Work out the finished part from the listing and answer in its coordinate system (mm). A direction names the side the tool comes from. Give positions to 0.01 mm unless a question says otherwise; leave off trailing zeros. Loops run counter-clockwise (first coordinate to the right, second up) from the corner with the lowest first, then second, coordinate; pieces in that order, holes last.
```python
from build123d import *

# Parameters (mm, degrees)
RESSALTO_EXTRUS_O2_DEPTH = 30
ESBO_O5_R                = 6
CORTE_EXTRUS_O1_DEPTH    = 30


with BuildPart() as part:
    # Esboço3 → Ressalto-extrusão2 (new body)
    with BuildSketch(Plane(origin=(0, 0, 0), x_dir=(0, 0, -1), z_dir=(1, 0, 0))):
        with BuildLine():
            Line((42.248831229, -47.335013165), (42.248831229, 2.664986835))
            Line((42.248831229, 2.664986835), (32.248831229, 2.664986835))
            Line((32.248831229, 2.664986835), (32.248831229, -1.335013165))
            ThreePointArc((32.248831229, -1.335013165), (30.491471916, -5.577653852), (26.248831229, -7.335013165))
            Line((26.248831229, -7.335013165), (6.748831229, -7.335013165))
            ThreePointArc((6.748831229, -7.335013165), (-3.504217098, -11.581964838), (-7.751168771, -21.835013165))
            Line((-7.751168771, -21.835013165), (-7.751168771, -22.835013165))
            ThreePointArc((-7.751168771, -22.835013165), (-3.504217098, -33.088061493), (6.748831229, -37.335013165))
            Line((6.748831229, -37.335013165), (26.248831229, -37.335013165))
            ThreePointArc((26.248831229, -37.335013165), (30.491471916, -39.092372478), (32.248831229, -43.335013165))
            Line((32.248831229, -43.335013165), (32.248831229, -47.335013165))
            Line((32.248831229, -47.335013165), (42.248831229, -47.335013165))
        make_face()
    extrude(amount=-RESSALTO_EXTRUS_O2_DEPTH)

    # Esboço5 → Corte-extrusão1 (cut)
    with BuildSketch(Plane(origin=(0, 0, 0), x_dir=(0, 0, -1), z_dir=(1, 0, 0))):
        with Locations((6.748831229, -22.335013165)):
            Circle(ESBO_O5_R)
    extrude(amount=-CORTE_EXTRUS_O1_DEPTH, mode=Mode.SUBTRACT)


solid = part.part
```
Q1. Section C-C on x = -21 is taken. Give the vertices of the cut face in (y, z), plus the area to 3 significant figures.
Q2. Which of the six approach directions +Z, -Z, +X, -X, +Y, -Y give full straight-line access (tool end or side, diameter ignored) to faces 1 (the face through (-15, 1, -32.249)), 2 (the face through (-15, -23, -42.249)), 3 (the face through (-15, -45, -32.249))?
Q3. Section B-B on y = -17 is taken. Give the vertices of the cut face in (x, z).
Q4. Section D-D on z = -24 is taken. Give the vertices of the cut face in (x, y).
Q5. Section A-A on z = -4 is taken. Give the vertices of the cut face in (x, y), plus the area to 3 significant figures.
Q6. Given pin 1 (15.5 mm diameter, centred on x = -12.5, z = -20.5, fed in from +Y); pin 2 (2 mm diameter, centred on x = -5, z = -1.5, fed in from +Y); pin 3 (15.5 mm diameter, centred on x = -11, z = -18.5, fed in from -Y) (3 decimals), each flat-ended and moving along its own axis, determine where each tip first touches the part or whether it passes through.
Q7. Consider line 1 along Y through (x, z) = (-1.5, -9); line 2 along Y through (x, z) = (-8, -8.5); line 3 along Y through (x, z) = (-7, -20). Determine where each line is inside the solid, lowest interval first.
Q8. Determine the mould class of faces 4 (the face through (-15, -47.335, -37)), 5 (the face through (-30, -22, -22)), 6 (the face through (-15, -7.335, -17)), 7 (the face through (-14.79, -17.276, -9.974)) for opening direction Y: +Y half, -Y half, draft (parallel to the pull), parting line (faces both ways), or undercut.
Check result:
1. outline: (-47.34, -42.25) - (2.66, -42.25) - (2.66, -32.25) - (-1.34, -32.25) arc R6 cw to (-7.34, -26.25) - (-7.34, -6.75) arc R14.5 ccw to (-21.84, 7.75) - (-22.84, 7.75) arc R14.5 ccw to (-37.34, -6.75) - (-37.34, -26.25) arc R6 cw to (-43.34, -32.25) - (-47.34, -32.25) - close; hole circle Ø12 at (-22.34, -6.75)
1. area: 1,510 mm2
2. face 1: +Z, +X, -X, +Y
2. face 2: -Z, +X, -X, +Y, -Y
2. face 3: +Z, +X, -X, -Y
3. outline: (-30, -42.25) - (0, -42.25) - (0, -9.49) - (-30, -9.49) - close; (-30, -4) - (0, -4) - (0, 6.92) - (-30, 6.92) - close
4. outline: (-30, -37.34) - (0, -37.34) - (0, -7.34) - (-30, -7.34) - close
5. outline: (-30, -37.07) - (0, -37.07) - (0, -27.67) - (-30, -27.67) - close; (-30, -17) - (0, -17) - (0, -7.6) - (-30, -7.6) - close
5. area: 564 mm2
6. pin 1: stops at y = -6.99
6. pin 2: stops at y = -7.97
6. pin 3: stops at y = -37.335
7. line 1: y = -37.34 to -27.9, -16.77 to -7.34
7. line 2: y = -37.34 to -28.07, -16.6 to -7.34
7. line 3: y = -37.34 to -7.34
8. face 4: -Y half
8. face 5: draft
8. face 6: +Y half
8. face 7: undercut
